Here's how the part is built. I have some questions about the finished solid (model axes, mm). Round coordinates to 2 decimals unless told otherwise and drop trailing zeros. Write each loop counter-clockwise with the first axis right and the second up, starting at its lowest first coordinate (ties: lowest second). Pieces come first, ordered by that corner, then holes. Notation, with made-up numbers: (2.25, 23) - (49.25, 23) arc R35 ccw to (49.25, 59) - close; hole circle Ø4 at (38, 77). An arc over 180 degrees is marked (long way). Write item = value, one per line. Start each with the question number.
Item 1: If I drill on line 1 along X through (y, z) = (6.7, -180); line 2 along X through (y, z) = (3, -60); line 3 along X through (y, z) = (2.25, 167), over which ranges is the centre line in solid material (lowest first)? Write a range as [from, to].
Item 2: If we section it at A-A (z = -26.5): Please give me the cut outline in (x, y) (3 decimals), and give its area (3 significant figures).
Item 3: For P1, Ø0.6, axis at x = 0, z = 211, coming from the -Y side; P2, Ø1, axis at y = 4, z = -167.5, coming from the +X side; P3, Ø2, axis at y = 9, z = -75.5, coming from the -X side, each with a flat end and sliding along its axis, tell me the tip position at first contact or that it passes through.
```python
from build123d import *

# Parameters (mm, degrees)
EXTRUDE_2_DEPTH        = 250
SKETCH_4_R             = 2.25
CUT_EXTRUDE_2_DEPTH    = 251.561868607
SKETCH_5_R             = 3.75
CUT_EXTRUDE_3_DEPTH    = 5.3
PATTERN_LINEAR_1_COUNT = 9
PATTERN_LINEAR_1_PITCH = 60


with BuildPart() as part:
    # 草图1 → 凸台-拉伸2 (new, symmetric)
    with BuildSketch(Plane.XY):
        with BuildLine():
            Line((6.75, 8.404656305), (6.205141704, 9.238414341))
            ThreePointArc((6.205141704, 9.238414341), (5.686086188, 9.347186448), (5.794858296, 9.866241964))
            Line((5.794858296, 9.866241964), (5.25, 10.7))
            Line((5.25, 10.7), (-5.25, 10.7))
            Line((-5.25, 10.7), (-5.794858296, 9.866241964))
            ThreePointArc((-5.794858296, 9.866241964), (-5.686086188, 9.347186448), (-6.205141704, 9.238414341))
            Line((-6.205141704, 9.238414341), (-6.75, 8.404656305))
            Line((-6.75, 8.404656305), (-6.75, 6.293987085))
            Line((-6.75, 6.293987085), (-6.023522272, 5.612625848))
            ThreePointArc((-6.023522272, 5.612625848), (-5.493464298, 5.629612418), (-5.476477728, 5.099554443))
            Line((-5.476477728, 5.099554443), (-4.75, 4.418193206))
            Line((-4.75, 4.418193206), (-4.75, 2.307523986))
            Line((-4.75, 2.307523986), (-7.5, 0))
            Line((-7.5, 0), (-7.5, -3.8))
            Line((-7.5, -3.8), (-7, -4.3))
            Line((-7, -4.3), (-1.5, -4.3))
            Line((-1.5, -4.3), (-1, -3.8))
            Line((-1, -3.8), (1, -3.8))
            Line((1, -3.8), (1.5, -4.3))
            Line((1.5, -4.3), (7, -4.3))
            Line((7, -4.3), (7.5, -3.8))
            Line((7.5, -3.8), (7.5, 0))
            Line((7.5, 0), (4.75, 2.307523986))
            Line((4.75, 2.307523986), (4.75, 4.418193206))
            Line((4.75, 4.418193206), (5.476477728, 5.099554443))
            ThreePointArc((5.476477728, 5.099554443), (5.493464298, 5.629612418), (6.023522272, 5.612625848))
            Line((6.023522272, 5.612625848), (6.75, 6.293987085))
            Line((6.75, 6.293987085), (6.75, 8.404656305))
        make_face()
    extrude(amount=EXTRUDE_2_DEPTH, both=True)

    # 草图4 → 切除-拉伸2 (cut, through all)
    with BuildSketch(Plane(origin=(0, 10.7, 0), x_dir=(1, 0, 0), z_dir=(0, 1, 0))):
        with Locations(Location((0, -240, 0), (0, 0, 270))):
            Circle(SKETCH_4_R)
    cut_extrude_2 = extrude(amount=-CUT_EXTRUDE_2_DEPTH, mode=Mode.SUBTRACT)

    # 草图5 → 切除-拉伸3 (cut)
    with BuildSketch(Plane(origin=(0, 10.7, 0), x_dir=(1, 0, 0), z_dir=(0, 1, 0))):
        with Locations(Location((0, -240, 0), (0, 0, 270))):
            Circle(SKETCH_5_R)
    cut_extrude_3 = extrude(amount=-CUT_EXTRUDE_3_DEPTH, mode=Mode.SUBTRACT)

    # 阵列(线性)1: 切除-拉伸2, 切除-拉伸3 ×9
    with Locations(*[(0, 0, -i * PATTERN_LINEAR_1_PITCH) for i in range(1, PATTERN_LINEAR_1_COUNT)]):
        add(cut_extrude_2, mode=Mode.SUBTRACT)
        add(cut_extrude_3, mode=Mode.SUBTRACT)


solid = part.part
```
Reply:
q1.line_1 = [-6.75, -3.75], [3.75, 6.75]
q1.line_2 = [-4.75, -2.25], [2.25, 4.75]
q1.line_3 = [-4.82, 4.82]
q2.outline = (-7.5, -3.8) - (-7, -4.3) - (-1.5, -4.3) - (-1, -3.8) - (1, -3.8) - (1.5, -4.3) - (7, -4.3) - (7.5, -3.8) - (7.5, 0) - (4.75, 2.308) - (4.75, 4.418) - (5.476, 5.1) arc R0.375 cw to (6.024, 5.613) - (6.75, 6.294) - (6.75, 8.405) - (6.205, 9.238) arc R0.375 cw to (5.795, 9.866) - (5.25, 10.7) - (-5.25, 10.7) - (-5.795, 9.866) arc R0.375 cw to (-6.205, 9.238) - (-6.75, 8.405) - (-6.75, 6.294) - (-6.024, 5.613) arc R0.375 cw to (-5.476, 5.1) - (-4.75, 4.418) - (-4.75, 2.308) - (-7.5, 0) - close
q2.area = 188 mm2
q3.P1 = -3.8
q3.P2 = 4.84
q3.P3 = -6.75
